Work out the finished part from the listing and answer in its coordinate system (mm). A direction names the side the tool comes from. Give positions to 0.01 mm unless a question says otherwise; leave off trailing zeros. Order: outer loops, then holes, each group sorted by start corner. A loop starts at its lowest first (then second) coordinate and runs counter-clockwise, first axis right, second up.
```python
from build123d import *

# Parameters (mm, degrees)
F0_R     = 45
F1_DEPTH = 25
F2_R     = 32.5
F3_DEPTH = 10
F5_R     = 35
F5_R_2   = 32.5
F6_DEPTH = 5


with BuildPart() as f1:
    # F0 (on Front) → F1 (new body)
    with BuildSketch(Plane.XZ):
        Circle(F0_R)
    extrude(amount=F1_DEPTH)

    # F2 (on face) → F3 (cut)
    with BuildSketch(Plane.XZ.offset(25)):
        Circle(F2_R)
    extrude(amount=-F3_DEPTH, mode=Mode.SUBTRACT)

    # F5 (on offset) → F6 (cut)
    with BuildSketch(Plane.XZ.offset(20)):
        Circle(F5_R)
        Circle(F5_R_2, mode=Mode.SUBTRACT)
    extrude(amount=-F6_DEPTH, mode=Mode.SUBTRACT)


solid = f1.part
```
1. Straight lines are drawn through the part: probe 1 along Y at (x, z) = (-22.5, -26.5); probe 2 along Z at (x, y) = (0.5, -16.25); probe 3 along Y at (x, z) = (12, 2.5). For each, find the intervals that lie inside material, in ascending order.
Findings below:
probe 1: y = -25 to -20, -15 to 0
probe 2: z = -45 to -35, 35 to 45
probe 3: y = -15 to 0
2. The mould has two halves that part along X. Classify faces 1 (the face through (23.2, -20, -23.2)), 2 (the face through (20.765, -12.325, -39.923)), 3 (the face through (-1, 0, 1)), 4 (the face through (-28, -18, -21)): pulls with the +X half, pulls with the -X half, needs draft (parallel to the pull), parting line crosses it, or undercut.
Findings below:
face 1: undercut
face 2: parting line crosses it
face 3: needs draft
face 4: undercut
3. The part is cut by section D-D (x = -38.5). Write down the section's boundary in (y, z), then the cut area to 3 significant figures.
Findings below:
outline: (-25, -23.3) - (0, -23.3) - (0, 23.3) - (-25, 23.3) - close
area: 1,160 mm2
4. The part is cut by section B-B (x = 0). Write down the section's boundary in (y, z).
Findings below:
outline: (-25, -45) - (0, -45) - (0, 45) - (-25, 45) - (-25, 32.5) - (-20, 32.5) - (-20, 35) - (-15, 35) - (-15, -35) - (-20, -35) - (-20, -32.5) - (-25, -32.5) - close
5. The part is cut by section A-A (z = 0). Write down the section's boundary in (x, y).
Findings below:
outline: (-45, -25) - (-32.5, -25) - (-32.5, -20) - (-35, -20) - (-35, -15) - (35, -15) - (35, -20) - (32.5, -20) - (32.5, -25) - (45, -25) - (45, 0) - (-45, 0) - close
6. Given P1, Ø2, axis at x = 1, y = -5, coming from the +Z side; P2, Ø5, axis at y = -21, z = 4.5, coming from the -X side; P3, Ø2, axis at x = -20.5, y = -9, coming from the +Z side; P4, Ø21, axis at x = 10, z = -4.5, coming from the +Y side, each flat-ended and moving along its own axis, determine where each tip first touches the part or whether it passes through.
Findings below:
P1: stops at z = 45
P2: stops at x = -44.96
P3: stops at z = 40.56
P4: stops at y = 0
7. The part is cut by section C-C (y = -7.75). Write down the section's boundary in (x, z).
Findings below:
outline: circle Ø90 at (0, 0)
8. Which of the six approach directions +Z, -Z, +X, -X, +Y, -Y give full straight-line access (tool end or side, diameter ignored) to faces 5 (the face through (13, -25, -30)), 6 (the face through (0, -15, 0)), 7 (the face through (31, -22.54, 9.76))?
Findings below:
face 5: +Z, -Z, +X, -X, -Y
face 6: none
face 7: -Y
